Autodesk Inventor part; units mm, degrees
ref_plane "YZ Plane" through (0, 0, 0) normal (1, 0, 0) x (0, 1, 0)
ref_plane "XZ Plane" through (0, 0, 0) normal (0, 1, 0) x (-1, 0, 0)
ref_plane "XY Plane" through (0, 0, 0) normal (0, 0, 1) x (1, 0, 0)
sketch "Sketch1" plane through (0, 0, 0) normal (0, 1, 0) x (-1, 0, 0)
  circle A0 centre (0, 0) radius 20
  dimension "d0" = 40
extrude "Extrusion1" add sketch "Sketch1" along normal blind 6
sketch "Sketch2" plane through (0, 6, 0) normal (0, 1, 0) x (1, 0, 0)
  circle A0 centre (0, 0) radius 17.5
  dimension "d3" = 35
extrude "Extrusion2" add sketch "Sketch2" along normal blind 6.8
sketch "Sketch3" plane through (0, 12.8, 0) normal (0, 1, 0) x (1, 0, 0)
  circle A0 centre (0, 0) radius 14.5 construction
  line L0 (0, 0) -> (-14.5, 0) construction
  point P0 (7.25, -12.5574)
  point P1 (7.25, 12.5574)
  dimension "d6" = 29
  dimension "d9" = 360
hole "Hole1" at (-14.5, 12.8, 0) at (7.25, 12.8, 12.5574) at (7.25, 12.8, -12.5574) direction (0, -1, 0) diameter 4.3 end through all
properties part number "Arm - slew column B"
Read the model definition and answer for the solid it produces. Units are mm, in the model's axes. A direction names the side the tool comes from. Give positions to 0.01 mm unless a question says otherwise; leave off trailing zeros. Loops run counter-clockwise (first coordinate to the right, second up) from the corner with the lowest first, then second, coordinate; pieces in that order, holes last.
Item 1: Find the intervals of material crossed by line 1 along X through (y, z) = (7.5, 0); line 2 along Z through (x, y) = (5.5, 12.25); line 3 along Z through (x, y) = (0, 10), in increasing order.
Item 2: For faces 4 (the cylindrical face through (-13.887, 9.352, -10.648)), 5 (the cylindrical face through (6.6, 6.31, -10.51)), determine the directions among +Z, -Z, +X, -X, +Y, -Y from which every point of the face is accessible in a straight line to the end or side of a thin tool.
Item 3: The part is cut by section A-A (z = 11). Write down the section's boundary in (x, y), and give its area (3 significant figures).
Item 4: The part is cut by section B-B (x = 7.25). Write down the section's boundary in (y, z), and give its area (3 significant figures).
Item 5: The part is cut by section D-D (x = -14.5). Write down the section's boundary in (y, z).
Item 6: The mould has two halves that part along Z. Classify faces 1 (the cylindrical face through (-12.4, 6.31, -0.47)), 2 (the cylindrical face through (4.336, 2.958, 19.524)), 3 (the flat face through (0, 12.8, 0)): released by +Z, released by -Z, zero draft, split by the parting line, or undercut.
Item 7: Each of these flat-tipped pins is pushed along its axis until it touches: pin 1 Ø2 at (y, z) = (3.5, 13.5) entering from -X; pin 2 Ø2 at (x, y) = (0, 1.5) entering from -Z; pin 3 Ø4 at (y, z) = (9.5, -9.5) entering from +X. Where does it stop, or does it pass through?
Item 8: The part is cut by section C-C (x = 0). Write down the section's boundary in (y, z), and give its area (3 significant figures).
Taken from the geometry:
1. line 1: x = -17.5 to -16.65, -12.35 to 17.5
1. line 2: z = -16.61 to -13.81, -11.31 to 11.31, 13.81 to 16.61
1. line 3: z = -17.5 to 17.5
2. face 4: +Y
2. face 5: +Y, -Y
3. outline: (-16.7, 0) - (5.77, 0) - (5.77, 12.8) - (-13.61, 12.8) - (-13.61, 6) - (-16.7, 6) - close; (8.73, 0) - (16.7, 0) - (16.7, 6) - (13.61, 6) - (13.61, 12.8) - (8.73, 12.8) - close
3. area: 348 mm2
4. outline: (0, -18.64) - (6, -18.64) - (6, -15.93) - (12.8, -15.93) - (12.8, -14.71) - (0, -14.71) - close; (0, -10.41) - (12.8, -10.41) - (12.8, 10.41) - (0, 10.41) - close; (0, 14.71) - (12.8, 14.71) - (12.8, 15.93) - (6, 15.93) - (6, 18.64) - (0, 18.64) - close
4. area: 330 mm2
5. outline: (0, -13.77) - (6, -13.77) - (6, -9.8) - (12.8, -9.8) - (12.8, -2.15) - (0, -2.15) - close; (0, 2.15) - (12.8, 2.15) - (12.8, 9.8) - (6, 9.8) - (6, 13.77) - (0, 13.77) - close
6. face 1: undercut
6. face 2: split by the parting line
6. face 3: zero draft
7. pin 1: stops at x = -15.61
7. pin 2: stops at z = -20
7. pin 3: stops at x = 15.81
8. outline: (0, -20) - (6, -20) - (6, -17.5) - (12.8, -17.5) - (12.8, 17.5) - (6, 17.5) - (6, 20) - (0, 20) - close
8. area: 478 mm2
